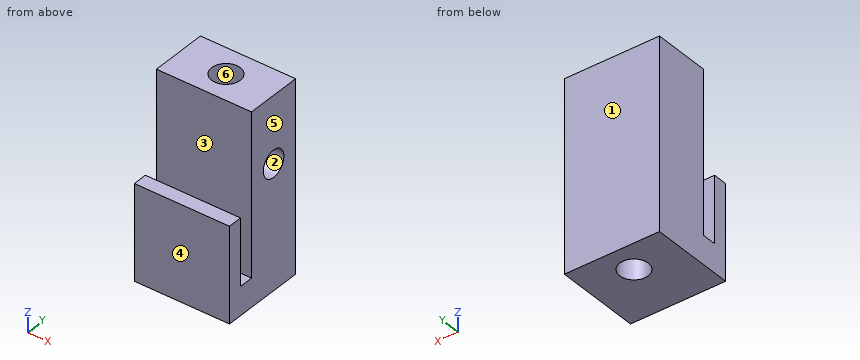
from build123d import *

# Parameters (mm, degrees)
SKETCH_W        = 10
SKETCH_H        = 6
PAD_DEPTH       = 20
SKETCH001_R     = 1.5
POCKET_DEPTH    = 20.001
SKETCH002_W     = 10
SKETCH002_H     = 0.01
POCKET001_DEPTH = 20.001
SKETCH003_W     = 10
SKETCH003_H     = 10
PAD001_DEPTH    = 3
SKETCH004_W     = 1.5
SKETCH004_H     = 7
POCKET002_DEPTH = 10.001
SKETCH005_R     = 1.4
POCKET003_DEPTH = 5


with BuildPart() as part:
    # Sketch → Pad (new body)
    with BuildSketch(Plane.XY):
        Rectangle(SKETCH_W, SKETCH_H)
    extrude(amount=PAD_DEPTH)

    # Sketch001 (on Face6 of Pad) → Pocket (cut, through all)
    with BuildSketch(Plane.XY.offset(20)):
        Circle(SKETCH001_R)
    extrude(amount=-POCKET_DEPTH, mode=Mode.SUBTRACT)

    # Sketch002 (on Face5 of Pocket) → Pocket001 (cut, through all)
    with BuildSketch(Plane.XY.offset(20)):
        with Locations((0, 3.005)):
            Rectangle(SKETCH002_W, SKETCH002_H)
    extrude(amount=-POCKET001_DEPTH, mode=Mode.SUBTRACT)

    # Sketch003 (on Face1 of Pocket001) → Pad001 (join)
    with BuildSketch(Plane.XZ.offset(3)):
        with Locations((0, 5)):
            Rectangle(SKETCH003_W, SKETCH003_H)
    extrude(amount=PAD001_DEPTH)

    # Sketch004 (on Face6 of Pad001) → Pocket002 (cut, through all)
    with BuildSketch(Plane.YZ.offset(5)):
        with Locations((-3.75, 6.5)):
            Rectangle(SKETCH004_W, SKETCH004_H)
    extrude(amount=-POCKET002_DEPTH, mode=Mode.SUBTRACT)

    # Sketch005 (on Face3 of Pocket002) → Pocket003 (cut)
    with BuildSketch(Plane.YZ.offset(5)):
        with Locations((0, 13)):
            Circle(SKETCH005_R)
    extrude(amount=-POCKET003_DEPTH, mode=Mode.SUBTRACT)


solid = part.part
Model file for the job. Use its own axes, mm. Face numbers are marked on the shaded views. A direction names the side the tool comes from. Round coordinates to 2 decimals unless told otherwise and drop trailing zeros. Order: outer loops, then holes, each group sorted by start corner. A loop starts at its lowest first (then second) coordinate and runs counter-clockwise, first axis right, second up.
(1) Band-saw the part on D-D (x = -2.5). List the corners of the cut face in (y, z).
(2) Band-saw the part on B-B (y = 0). List the corners of the cut face in (x, z), then the cut area to 3 significant figures.
(3) Pull direction Y, two halves, no side cores. Call the marked faces 4, 5 and 6: released by +Y, released by -Y, zero draft, split by the parting line, or undercut.
(4) Pin check, flat tips, straight feed: pin 1 (1.7 mm diameter, centred on y = 0, z = 13, fed in from +X); pin 2 (5 mm diameter, centred on x = 3, y = -3, fed in from -Z); pin 3 (1.2 mm diameter, centred on x = -1.5, y = -5, fed in from +Z); pin 4 (4 mm diameter, centred on x = -1.5, z = 16, fed in from -Y). Stop position of each tip, or through.
(5) 3-axis set-ups, long thin cutter, end or side, ignore diameter. For the marked faces 1, 2 and 3: which of +Z, -Z, +X, -X, +Y, -Y reach the whole face in a straight line?
(6) Drill centre lines: line 1 (Y direction, x = 0, z = 6); line 2 (Z direction, x = 3.8, y = 0); line 3 (Y direction, x = 0, z = 10.75). Where is each one in solid material? Low to high.
(7) Band-saw the part on A-A (x = 0). List the corners of the cut face in (y, z).
(8) Band-saw the part on C-C (z = 2.25). List the corners of the cut face in (x, y), then the cut area to 3 significant figures.
Verdict:
1. outline: (-6, 0) - (3, 0) - (3, 20) - (-3, 20) - (-3, 3) - (-4.5, 3) - (-4.5, 10) - (-6, 10) - close
2. outline: (-5, 0) - (-1.5, 0) - (-1.5, 20) - (-5, 20) - close; (1.5, 0) - (5, 0) - (5, 11.6) - (1.5, 11.6) - close; (1.5, 14.4) - (5, 14.4) - (5, 20) - (1.5, 20) - close
2. area: 130 mm2
3. face 4: released by -Y
3. face 5: zero draft
3. face 6: undercut
4. pin 1: stops at x = -1.24
4. pin 2: stops at z = 0
4. pin 3: stops at z = 10
4. pin 4: stops at y = -3
5. face 1: +Z, -Z, +X, -X, +Y
5. face 2: +X
5. face 3: +Z, +X, -X
6. line 1: y = -6 to -4.5, -3 to -1.5, 1.5 to 3
6. line 2: z = 0 to 11.6, 14.4 to 20
6. line 3: y = -3 to -1.5, 1.5 to 3
7. outline: (-6, 0) - (-1.5, 0) - (-1.5, 20) - (-3, 20) - (-3, 3) - (-4.5, 3) - (-4.5, 10) - (-6, 10) - close; (1.5, 0) - (3, 0) - (3, 20) - (1.5, 20) - close
8. outline: (-5, -6) - (5, -6) - (5, 3) - (-5, 3) - close; hole circle Ø3 at (0, 0)
8. area: 82.9 mm2
